from build123d import *

# Parameters (mm, degrees)
BOSS_EXTRUDE1_DEPTH = 711.2
BOSS_EXTRUDE2_REACH = 963.601
SKETCH2_W           = 12.7
SKETCH2_H           = 2.54
SKETCH3_W           = 152.4
SKETCH3_H           = 609.6
SKETCH3_W_2         = 95.25
SKETCH3_W_3         = 12.7
CUT_EXTRUDE1_DEPTH  = 2.54
SKETCH4_W           = 12.7
SKETCH4_H           = 6.35
SKETCH4_H_2         = 2.54
BOSS_EXTRUDE3_DEPTH = 589.28
SKETCH5_W           = 571.5
SKETCH5_H           = 12.668198963
BOSS_EXTRUDE4_DEPTH = 2.54
BOSS_EXTRUDE5_START = -2.54
BOSS_EXTRUDE5_DEPTH = 2.54
SKETCH7_W           = 571.5
SKETCH7_H           = 19.05
BOSS_EXTRUDE6_DEPTH = 2.54
SKETCH9_W           = 571.5
SKETCH9_H           = 2.54
BOSS_EXTRUDE7_DEPTH = 69.85
SKETCH10_W          = 571.5
SKETCH10_H          = 22.86
BOSS_EXTRUDE8_DEPTH = 2.54
BOSS_EXTRUDE9_START = 10.16
BOSS_EXTRUDE9_DEPTH = 10.16


with BuildPart() as part:
    # Sketch1 → Boss-Extrude1 (new body)
    with BuildSketch(Plane(origin=(0, 0, 0), x_dir=(1, 0, 0), z_dir=(0, 1, 0))):
        with BuildLine():
            Line((-285.75, 175.26), (285.75, 175.26))
            ThreePointArc((285.75, 175.26), (301.914461018, 168.564461018), (308.61, 152.4))
            Line((308.61, 152.4), (308.61, -149.86))
            Line((308.61, -149.86), (285.75, -149.86))
            Line((285.75, -149.86), (285.75, -152.4))
            Line((285.75, -152.4), (311.15, -152.4))
            Line((311.15, -152.4), (311.15, 152.4))
            ThreePointArc((311.15, 152.4), (303.710512242, 170.360512242), (285.75, 177.8))
            Line((285.75, 177.8), (-285.75, 177.8))
            ThreePointArc((-285.75, 177.8), (-303.710512242, 170.360512242), (-311.15, 152.4))
            Line((-311.15, 152.4), (-311.15, -152.4))
            Line((-311.15, -152.4), (-285.75, -152.4))
            Line((-285.75, -152.4), (-285.75, -149.86))
            Line((-285.75, -149.86), (-308.61, -149.86))
            Line((-308.61, -149.86), (-308.61, 152.4))
            ThreePointArc((-308.61, 152.4), (-301.914461018, 168.564461018), (-285.75, 175.26))
        make_face()
    extrude(amount=BOSS_EXTRUDE1_DEPTH)

    # Boss-Extrude2: up to this face of the body (flat: up to its plane)
    boss_extrude2_end = Plane(part.part.faces().sort_by_distance((308.61, 355.6, -1.27))[0])
    # Sketch2 → Boss-Extrude2 (add, up to the picked face)
    with BuildSketch(Plane.ZY.offset(311.15), mode=Mode.PRIVATE) as boss_extrude2_sk1:
        Polygon((-100.33, 622.3), (-123.19, 622.3), (-123.19, 599.44), (-125.73, 599.44), (-125.73, 624.84), (-100.33, 624.84), align=None)
    boss_extrude2_tool1 = split(extrude(boss_extrude2_sk1.sketch, amount=-BOSS_EXTRUDE2_REACH, mode=Mode.PRIVATE), bisect_by=boss_extrude2_end, keep=Keep.BOTH, mode=Mode.PRIVATE)
    # Sketch2 → Boss-Extrude2 (add, up to the picked face)
    with BuildSketch(Plane.ZY.offset(311.15), mode=Mode.PRIVATE) as boss_extrude2_sk2:
        Polygon((58.42, 622.3), (35.56, 622.3), (35.56, 599.44), (29.21, 599.44), (29.21, 622.3), (6.35, 622.3), (6.35, 624.84), (58.42, 624.84), align=None)
    boss_extrude2_tool2 = split(extrude(boss_extrude2_sk2.sketch, amount=-BOSS_EXTRUDE2_REACH, mode=Mode.PRIVATE), bisect_by=boss_extrude2_end, keep=Keep.BOTH, mode=Mode.PRIVATE)
    # Sketch2 → Boss-Extrude2 (add, up to the picked face)
    with BuildSketch(Plane.ZY.offset(311.15), mode=Mode.PRIVATE) as boss_extrude2_sk3:
        Polygon((134.099064666, 599.44), (130.81, 599.44), (130.81, 622.3), (111.76, 622.3), (111.76, 624.84), (137.16, 624.84), (149.86, 624.84), (149.86, 622.3), (137.16, 622.3), (137.16, 599.44), align=None)
    boss_extrude2_tool3 = split(extrude(boss_extrude2_sk3.sketch, amount=-BOSS_EXTRUDE2_REACH, mode=Mode.PRIVATE), bisect_by=boss_extrude2_end, keep=Keep.BOTH, mode=Mode.PRIVATE)
    # Sketch2 → Boss-Extrude2 (add, up to the picked face)
    with BuildSketch(Plane.ZY.offset(311.15), mode=Mode.PRIVATE) as boss_extrude2_sk4:
        Polygon((-123.19, 35.56), (-123.19, 12.7), (-100.33, 12.7), (-100.33, 10.16), (-125.73, 10.16), (-125.73, 35.56), align=None)
    boss_extrude2_tool4 = split(extrude(boss_extrude2_sk4.sketch, amount=-BOSS_EXTRUDE2_REACH, mode=Mode.PRIVATE), bisect_by=boss_extrude2_end, keep=Keep.BOTH, mode=Mode.PRIVATE)
    # Sketch2 → Boss-Extrude2 (add, up to the picked face)
    with BuildSketch(Plane.ZY.offset(311.15), mode=Mode.PRIVATE) as boss_extrude2_sk5:
        Polygon((58.42, 12.7), (58.42, 10.16), (6.35, 10.16), (6.35, 12.7), (29.21, 12.7), (29.21, 35.56), (35.56, 35.56), (35.56, 12.7), align=None)
    boss_extrude2_tool5 = split(extrude(boss_extrude2_sk5.sketch, amount=-BOSS_EXTRUDE2_REACH, mode=Mode.PRIVATE), bisect_by=boss_extrude2_end, keep=Keep.BOTH, mode=Mode.PRIVATE)
    # Sketch2 → Boss-Extrude2 (add, up to the picked face)
    with BuildSketch(Plane.ZY.offset(311.15), mode=Mode.PRIVATE) as boss_extrude2_sk6:
        Polygon((137.16, 35.56), (137.16, 12.7), (137.16, 10.16), (111.76, 10.16), (111.76, 12.7), (130.81, 12.7), (130.81, 35.56), (134.099064666, 35.56), align=None)
    boss_extrude2_tool6 = split(extrude(boss_extrude2_sk6.sketch, amount=-BOSS_EXTRUDE2_REACH, mode=Mode.PRIVATE), bisect_by=boss_extrude2_end, keep=Keep.BOTH, mode=Mode.PRIVATE)
    # Sketch2 → Boss-Extrude2 (add, up to the picked face)
    with BuildSketch(Plane.ZY.offset(311.15), mode=Mode.PRIVATE) as boss_extrude2_sk7:
        with Locations((143.51, 11.43)):
            Rectangle(SKETCH2_W, SKETCH2_H)
    boss_extrude2_tool7 = split(extrude(boss_extrude2_sk7.sketch, amount=-BOSS_EXTRUDE2_REACH, mode=Mode.PRIVATE), bisect_by=boss_extrude2_end, keep=Keep.BOTH, mode=Mode.PRIVATE)
    add(boss_extrude2_tool1.solids().sort_by(Axis((-311.15, 622.65921, -111.76), (1, 0, 0)))[0])
    add(boss_extrude2_tool2.solids().sort_by(Axis((-311.15, 616.924651, 32.385), (1, 0, 0)))[0])
    add(boss_extrude2_tool3.solids().sort_by(Axis((-311.15, 615.95, 132.715), (1, 0, 0)))[0])
    add(boss_extrude2_tool4.solids().sort_by(Axis((-311.15, 24.13, -123.54921), (1, 0, 0)))[0])
    add(boss_extrude2_tool5.solids().sort_by(Axis((-311.15, 18.075349, 32.385), (1, 0, 0)))[0])
    add(boss_extrude2_tool6.solids().sort_by(Axis((-311.15, 20.222308, 131.054231), (1, 0, 0)))[0])
    add(boss_extrude2_tool7.solids().sort_by(Axis((-311.15, 11.43, 143.51), (1, 0, 0)))[0])

    # Sketch3 → Cut-Extrude1 (cut)
    with BuildSketch(Plane.ZY.offset(311.15)):
        with Locations((-46.99, 317.5)):
            Rectangle(SKETCH3_W, SKETCH3_H)
        with Locations((83.185, 317.5)):
            Rectangle(SKETCH3_W_2, SKETCH3_H)
        with Locations((143.51, 317.5)):
            Rectangle(SKETCH3_W_3, SKETCH3_H)
    extrude(amount=-CUT_EXTRUDE1_DEPTH, mode=Mode.SUBTRACT)

    # Sketch4 → Boss-Extrude3 (add)
    with BuildSketch(Plane(origin=(0, 624.84, 0), x_dir=(1, 0, 0), z_dir=(0, 1, 0))):
        with Locations((-302.26, -32.385)):
            Rectangle(SKETCH4_W, SKETCH4_H)
        with Locations((-302.26, -133.985)):
            Rectangle(SKETCH4_W, SKETCH4_H)
        with Locations((-302.26, 124.46)):
            Rectangle(SKETCH4_W, SKETCH4_H_2)
        with Locations((302.26, -133.985)):
            Rectangle(SKETCH4_W, SKETCH4_H)
        with Locations((302.26, -32.385)):
            Rectangle(SKETCH4_W, SKETCH4_H)
        with Locations((302.26, 124.46)):
            Rectangle(SKETCH4_W, SKETCH4_H_2)
    extrude(amount=-BOSS_EXTRUDE3_DEPTH)

    # Sketch5 → Boss-Extrude4 (add)
    with BuildSketch(Plane.XY.offset(152.4)):
        with Locations((0, 6.334099482)):
            Rectangle(SKETCH5_W, SKETCH5_H)
    extrude(amount=-BOSS_EXTRUDE4_DEPTH)

    # Sketch6 → Boss-Extrude5 (add)
    with BuildSketch(Plane(origin=(0, 711.2, 0), x_dir=(1, 0, 0), z_dir=(0, 1, 0)).offset(BOSS_EXTRUDE5_START)):
        with BuildLine():
            Line((-285.75, -149.86), (-285.75, -124.46))
            Line((-285.75, -124.46), (-285.75, 152.4))
            Line((-285.75, 152.4), (285.75, 152.4))
            Line((285.75, 152.4), (285.75, -127))
            Line((285.75, -127), (285.75, -149.86))
            Line((285.75, -149.86), (308.61, -149.86))
            Line((308.61, -149.86), (308.61, 152.4))
            ThreePointArc((308.61, 152.4), (301.914461018, 168.564461018), (285.75, 175.26))
            Line((285.75, 175.26), (-285.75, 175.26))
            ThreePointArc((-285.75, 175.26), (-301.914461018, 168.564461018), (-308.61, 152.4))
            Line((-308.61, 152.4), (-308.61, -149.86))
            Line((-308.61, -149.86), (-285.75, -149.86))
        make_face()
    extrude(amount=BOSS_EXTRUDE5_DEPTH)

    # Sketch7 → Boss-Extrude6 (add)
    with BuildSketch(Plane.XY.offset(149.86)):
        with Locations((0, 631.825)):
            Rectangle(SKETCH7_W, SKETCH7_H)
    extrude(amount=BOSS_EXTRUDE6_DEPTH)

    # Sketch9 → Boss-Extrude7 (add)
    with BuildSketch(Plane(origin=(0, 641.35, 0), x_dir=(1, 0, 0), z_dir=(0, 1, 0))):
        with Locations((0, -151.13)):
            Rectangle(SKETCH9_W, SKETCH9_H)
    extrude(amount=BOSS_EXTRUDE7_DEPTH)

    # Sketch10 → Boss-Extrude8 (add)
    with BuildSketch(Plane(origin=(0, 711.2, 0), x_dir=(1, 0, 0), z_dir=(0, 1, 0))):
        with Locations((0, -138.43)):
            Rectangle(SKETCH10_W, SKETCH10_H)
    extrude(amount=-BOSS_EXTRUDE8_DEPTH)

    # Sketch11 → Boss-Extrude9 (add)
    with BuildSketch(Plane.XZ.offset(-10.16).offset(BOSS_EXTRUDE9_START)):
        with BuildLine():
            Line((-308.61, 149.86), (-308.61, -152.4))
            ThreePointArc((-308.61, -152.4), (-301.914461018, -168.564461018), (-285.75, -175.26))
            Line((-285.75, -175.26), (285.75, -175.26))
            ThreePointArc((285.75, -175.26), (301.914461018, -168.564461018), (308.61, -152.4))
            Line((308.61, -152.4), (308.61, 149.86))
            Line((308.61, 149.86), (-308.61, 149.86))
        make_face()
    extrude(amount=-BOSS_EXTRUDE9_DEPTH)


solid = part.part
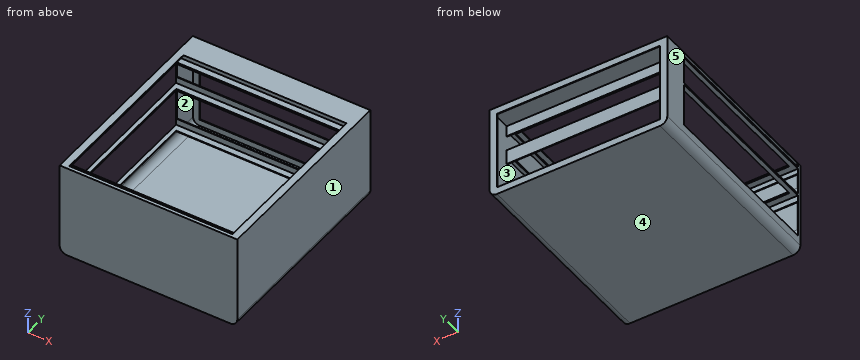
Verification items for the finished model (mm, model axes). Face numbers are marked on the shaded views. A direction names the side the tool comes from. Give positions to 0.01 mm unless a question says otherwise; leave off trailing zeros. Write each loop counter-clockwise with the first axis right and the second up, starting at its lowest first coordinate (ties: lowest second). Pieces come first, ordered by that corner, then holes.
(1) Material ranges on line 1 (Y direction, x = -248, z = 134.5); line 2 (Y direction, x = -228.5, z = -158); line 3 (Y direction, x = 62, z = 39), recorded low to high.
(2) Mould release check, pull along Z, two halves, no side actions. Record for the marked faces 3, 4 and 5: +Z half, -Z half, draft (parallel to the pull), parting line (faces both ways), or undercut.
(3) Cross-section at C-C (x = 183.5). State how many separate pieces and enclosed holes the cut face has, plus the area to 3 significant figures.
(4) Gauge pin test, flat ends, axial feed: pin 1 (4 mm diameter, centred on x = -198, z = 106.5, fed in from +Y); pin 2 (12 mm diameter, centred on x = -13.5, y = 170.5, fed in from +Z). Record the tip position at first contact, or that the pin passes through.
(5) Cross-section at B-B (z = 45). Enter the section's corners in (x, y).
(6) Access from +Z, -Z, +X, -X, +Y, -Y to the whole of each face (thin tool, end or side, straight path). Record for the marked faces 1 and 2.
(7) Cross-section at A-A (z = -46). Enter the section's corners in (x, y), plus the area to 3 significant figures.
Worked out:
1. line 1: y = 0 to 35.56, 599.44 to 624.84, 708.66 to 711.2
1. line 2: y = 0 to 10.16, 708.66 to 711.2
1. line 3: y = 0 to 12.7, 622.3 to 624.84
2. face 3: undercut
2. face 4: -Z half
2. face 5: draft
3. separate pieces: 4
3. enclosed holes: 0
3. area: 6,770 mm2
4. pin 1: stops at y = 10.16
4. pin 2: stops at z = -175.26
5. outline: (-311.15, 0) - (311.15, 0) - (311.15, 711.2) - (285.75, 711.2) - (285.75, 708.66) - (308.61, 708.66) - (308.61, 624.84) - (-308.61, 624.84) - (-308.61, 708.66) - (-285.75, 708.66) - (-285.75, 711.2) - (-311.15, 711.2) - (-311.15, 622.3) - (308.61, 622.3) - (308.61, 12.7) - (-311.15, 12.7) - close
6. face 1: +Z, -Z, +X, +Y, -Y
6. face 2: none
7. outline: (-311.15, 0) - (311.15, 0) - (311.15, 711.2) - (285.75, 711.2) - (285.75, 708.66) - (308.61, 708.66) - (308.61, 10.16) - (-308.61, 10.16) - (-308.61, 12.7) - (-311.15, 12.7) - close; (-311.15, 622.3) - (-308.61, 622.3) - (-308.61, 708.66) - (-285.75, 708.66) - (-285.75, 711.2) - (-311.15, 711.2) - close
7. area: 8,450 mm2
